```python
from build123d import *

# Parameters (mm, degrees)
F0_W     = 45
F0_H     = 18
F0_R     = 2.5
F1_DEPTH = 4
F2_R     = 3.75
F3_DEPTH = 10


with BuildPart() as f1:
    # F0 (on Top) → F1 (new body)
    with BuildSketch(Plane.XY):
        Rectangle(F0_W, F0_H)
        with Locations((-12.5, 0)):
            Circle(F0_R, mode=Mode.SUBTRACT)
        with Locations((12.5, 0)):
            Circle(F0_R, mode=Mode.SUBTRACT)
    extrude(amount=F1_DEPTH)

    # F2 (on face) → F3 (join)
    with BuildSketch(Plane.XY.offset(4)):
        Circle(F2_R)
    extrude(amount=F3_DEPTH)


solid = f1.part
```
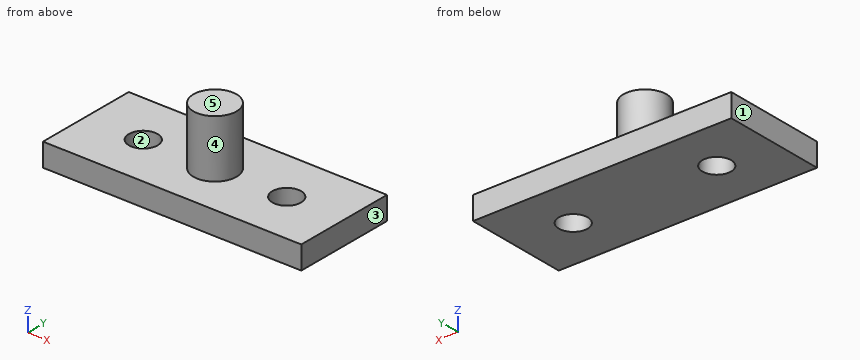
Here's how the part is built. I have some questions about the finished solid (model axes, mm). Face numbers are marked on the shaded views. A direction names the side the tool comes from. Give positions to 0.01 mm unless a question says otherwise; leave off trailing zeros. Write each loop counter-clockwise with the first axis right and the second up, starting at its lowest first coordinate (ties: lowest second). Pieces come first, ordered by that corner, then holes. Notation, with made-up numbers: (47.5, -21.75) -> (63.5, -21.75) arc R26 cw to (63.5, 5.25) -> close; hole circle Ø10 at (63, 1). An arc over 180 degrees is marked (long way). Write each question's results on one line, items separated by ' | '.
Item 1: Suppose I cut it at D-D on x = 0. Write out the boundary of the cut face in (y, z), plus the area to 3 significant figures.
Output:
outline: (-9, 0) -> (9, 0) -> (9, 4) -> (3.75, 4) -> (3.75, 14) -> (-3.75, 14) -> (-3.75, 4) -> (-9, 4) -> close | area: 147 mm^2
Item 2: For pin 1 Ø4.5 at (x, y) = (-12.5, 0) entering from -Z; pin 2 Ø6 at (x, y) = (12.5, 0) entering from +Z, each with a flat end and sliding along its axis, tell me the tip position at first contact or that it passes through.
Output:
pin 1: passes through | pin 2: stops at z = 4
Item 3: Suppose I cut it at C-C on z = 1.75. Write out the boundary of the cut face in (x, y).
Output:
outline: (-22.5, -9) -> (22.5, -9) -> (22.5, 9) -> (-22.5, 9) -> close; hole circle Ø5 at (-12.5, 0); hole circle Ø5 at (12.5, 0)
Item 4: We'd pull the mould along X, two halves only. Please class the marked faces 1, 2 and 3: pulls with the +X half, pulls with the -X half, needs draft (parallel to the pull), parting line crosses it, or undercut.
Output:
face 1: pulls with the -X half | face 2: undercut | face 3: pulls with the +X half
Item 5: Suppose I cut it at A-A on x = 14. Write out the boundary of the cut face in (y, z), plus the area to 3 significant figures.
Output:
outline: (-9, 0) -> (-2, 0) -> (-2, 4) -> (-9, 4) -> close; (2, 0) -> (9, 0) -> (9, 4) -> (2, 4) -> close | area: 56.0 mm^2
Item 6: If I drill on L1, parallel to Y at x = -12.5, z = 2.85; L2, parallel to Z at x = -14, y = -8; L3, parallel to Y at x = 11.5, z = 3.75, over which ranges is the centre line in solid material (lowest first)?
Output:
L1: y = -9 to -2.5, 2.5 to 9 | L2: z = 0 to 4 | L3: y = -9 to -2.29, 2.29 to 9
Item 7: On a 3-axis mill with a long thin cutter (end or side, diameter ignored), from which of +Z, -Z, +X, -X, +Y, -Y can I reach the whole of each face in a straight line? I mean the marked faces 4 and 5. Say none if no direction works.
Output:
face 4: +Z | face 5: +Z, +X, -X, +Y, -Y
Item 8: Suppose I cut it at B-B on y = 0. Write out the boundary of the cut face in (x, z).
Output:
outline: (-22.5, 0) -> (-15, 0) -> (-15, 4) -> (-22.5, 4) -> close; (-10, 0) -> (10, 0) -> (10, 4) -> (3.75, 4) -> (3.75, 14) -> (-3.75, 14) -> (-3.75, 4) -> (-10, 4) -> close; (15, 0) -> (22.5, 0) -> (22.5, 4) -> (15, 4) -> close
